from build123d import *

# Parameters (mm, degrees)
CROQUIS1_R                 = 8.24
SALIENTE_EXTRUIR1_DEPTH    = 6
CROQUIS3_R                 = 7.85
SALIENTE_EXTRUIR2_DEPTH    = 134.8
CROQUIS4_R                 = 4.835
CORTAR_EXTRUIR1_DEPTH      = 142.281404297
CORTAR_EXTRUIR2_DEPTH      = 142.281404297
CORTAR_EXTRUIR2_DEPTH_BACK = 142.281404297


with BuildPart() as part:
    # Croquis1 → Saliente-Extruir1 (new body)
    with BuildSketch(Plane(origin=(0, 0, 0), x_dir=(1, 0, 0), z_dir=(0, 1, 0))):
        with Locations(Location((0, 0, 0), (0, 0, 270))):
            Circle(CROQUIS1_R)
    extrude(amount=SALIENTE_EXTRUIR1_DEPTH)

    # Croquis2 → Cortar-Revolución1 (revolve, cut)
    with BuildSketch(Plane.XY, mode=Mode.PRIVATE) as cortar_revoluci_n1_sk:
        Polygon((-8.24, 0), (-7.883666073, 6), (-8.24, 6), align=None)
    revolve(cortar_revoluci_n1_sk.sketch.rotate(Axis((0, 0, 0), (0, 1, 0)), 270), axis=Axis((0, 0, 0), (0, 1, 0)), mode=Mode.SUBTRACT)

    # Croquis3 → Saliente-Extruir2 (add)
    with BuildSketch(Plane(origin=(0, 6, 0), x_dir=(1, 0, 0), z_dir=(0, 1, 0))):
        with Locations(Location((0, 0, 0), (0, 0, 270))):
            Circle(CROQUIS3_R)
    extrude(amount=SALIENTE_EXTRUIR2_DEPTH)

    # Croquis4 → Cortar-Extruir1 (cut, through all)
    with BuildSketch(Plane(origin=(0, 140.8, 0), x_dir=(1, 0, 0), z_dir=(0, 1, 0))):
        with Locations(Location((0, 0, 0), (0, 0, 270))):
            Circle(CROQUIS4_R)
    extrude(amount=-CORTAR_EXTRUIR1_DEPTH, mode=Mode.SUBTRACT)

    # Croquis5 → Cortar-Extruir2 (cut, two sides: drawn at the far end of the back side and taken through both)
    with BuildSketch(Plane.XY.offset(-CORTAR_EXTRUIR2_DEPTH_BACK)):
        with BuildLine():
            Line((1.65, 140.8), (-1.65, 140.8))
            Line((-1.65, 140.8), (-1.65, 11.621418712))
            ThreePointArc((-1.65, 11.621418712), (0, 9.97), (1.65, 11.621418712))
            Line((1.65, 11.621418712), (1.65, 140.8))
        make_face()
    extrude(amount=CORTAR_EXTRUIR2_DEPTH + CORTAR_EXTRUIR2_DEPTH_BACK, mode=Mode.SUBTRACT)

    # Croquis7 → Cortar-Revolución2 (revolve, cut)
    with BuildSketch(Plane.XY, mode=Mode.PRIVATE) as cortar_revoluci_n2_sk:
        Polygon((11.646495886, 140.8), (7.85, 133.06), (5.823247943, 140.8), align=None)
    revolve(cortar_revoluci_n2_sk.sketch.rotate(Axis((0, 140.8, 0), (0, -1, 0)), 257.866449584), axis=Axis((0, 140.8, 0), (0, -1, 0)), mode=Mode.SUBTRACT)


solid = part.part
Geometry check sheet. Reference: the model listing, model coordinates, mm. A direction names the side the tool comes from. Give positions to 0.01 mm unless a question says otherwise; leave off trailing zeros. Order: outer loops, then holes, each group sorted by start corner. A loop starts at its lowest first (then second) coordinate and runs counter-clockwise, first axis right, second up. Notation, with made-up numbers: M -23.5,16 L 1.5,16 A18 cw 1.5,22 Z; hole C 33,-26 d5. An arc over 180 degrees is marked long. Use a Markdown table: item, result.
Item 1: Section check C-C (x = 0). Record the cut outline in (y, z) (3 decimals), and give its area (3 significant figures).
Answers follow:
| item | result |
|---|---|
| outline | M 0,-8.24 L 6,-7.884 L 6,-7.85 L 9.97,-7.85 L 9.97,-4.835 L 0,-4.835 Z; M 0,4.835 L 9.97,4.835 L 9.97,7.85 L 6,7.85 L 6,7.884 L 0,8.24 Z |
| area | 62.7 mm2 |
Item 2: Depth check by flat-ended pin: P1, Ø3.5, axis at y = 72, z = 6.5, coming from the -X side; P2, Ø8, axis at y = 50, z = 1, coming from the -X side; P3, Ø2.5, axis at y = 92, z = -7, coming from the +X side; P4, Ø2, axis at x = 4.5, z = 0.5, coming from the -Y side. Enter the tip coordinate at first touch or a pass-through.
Answers follow:
| item | result |
|---|---|
| P1 | stops at x = -6.25 |
| P2 | stops at x = -7.85 |
| P3 | stops at x = 5.34 |
| P4 | stops at y = 0 |
Item 3: Material ranges on line 1 along X through (y, z) = (27, -5.25); line 2 along X through (y, z) = (88, 0) (3 decimals); line 3 along Z through (x, y) = (-3, 79.5), recorded low to high.
Answers follow:
| item | result |
|---|---|
| line 1 | x = -5.84 to -1.65, 1.65 to 5.84 |
| line 2 | x = -7.85 to -4.835, 4.835 to 7.85 |
| line 3 | z = -7.25 to -3.79, 3.79 to 7.25 |
Item 4: Tool access check on faces 1 (the cylindrical face through (-3.01, 68.64, 7.25)), 2 (the flat face through (-1.65, 77, 6)), 3 (the flat face through (-4, 0, 4)). Record the directions out of +Z, -Z, +X, -X, +Y, -Y that give a thin tool (end or side, any length) a straight path to the whole face; none if there is none.
Answers follow:
| item | result |
|---|---|
| face 1 | +Y |
| face 2 | +Z, -Z, +Y |
| face 3 | +Z, -Z, +X, -X, -Y |
Item 5: Draft check along X on faces 4 (the conical face through (4.88, 3.709, 6.364)), 5 (the cylindrical face through (-4.72, 71.39, -1.05)), 6 (the cylindrical face through (-0.04, 9.97, -6.22)), 7 (the flat face through (5, 140.8, 0)). Enter one of: +X half, -X half, draft (parallel to the pull), parting line (faces both ways), or undercut.
Answers follow:
| item | result |
|---|---|
| face 4 | parting line |
| face 5 | undercut |
| face 6 | undercut |
| face 7 | draft |
Item 6: Section check B-B (z = 0). Record the cut outline in (x, y) (3 decimals).
Answers follow:
| item | result |
|---|---|
| outline | M -8.24,0 L -4.835,0 L -4.835,140.8 L -5.823,140.8 L -7.85,133.06 L -7.85,6 L -7.884,6 Z; M 4.835,0 L 8.24,0 L 7.884,6 L 7.85,6 L 7.85,133.06 L 5.823,140.8 L 4.835,140.8 Z |
Item 7: Section check A-A (y = 46). Record the cut outline in (x, z) (3 decimals).
Answers follow:
| item | result |
|---|---|
| outline | M -1.65,-7.675 L -1.65,-4.545 A4.835 cw -1.65,4.545 L -1.65,7.675 A7.85 ccw Z; M 1.65,-7.675 A7.85 ccw 1.65,7.675 L 1.65,4.545 A4.835 cw 1.65,-4.545 Z |
